Check sheet for the modelled part. Datum: model origin and axes. Units: mm. Face numbers are marked on the shaded views. Round coordinates to 2 decimals unless told otherwise and drop trailing zeros. Order: outer loops, then holes, each group sorted by start corner. A loop starts at its lowest first (then second) coordinate and runs counter-clockwise, first axis right, second up. Notation, with made-up numbers: (-39.5, -27.5) -> (15.5, -27.5) arc R16 ccw to (15.5, -2.5) -> close; hole circle Ø2 at (88.25, -34). An arc over 180 degrees is marked (long way). Use CSV: the item, a comma, the result in double quotes.
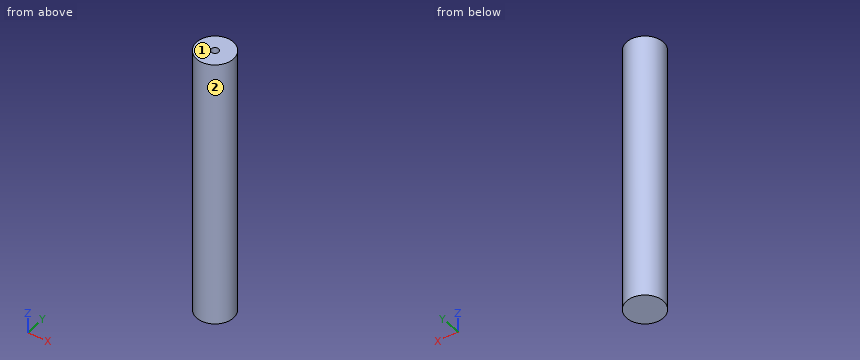
```python
from build123d import *

# Parameters (mm, degrees)
SKETCH009_R     = 5
PAD006_DEPTH    = 74
SKETCH010_R     = 1
POCKET002_DEPTH = 5
SKETCH011_R     = 1
POCKET003_DEPTH = 5


with BuildPart() as part:
    # Sketch009 → Pad006 (new body)
    with BuildSketch(Plane.XY):
        Circle(SKETCH009_R)
    extrude(amount=PAD006_DEPTH)

    # Sketch010 → Pocket002 (cut)
    with BuildSketch(Plane.XY):
        Circle(SKETCH010_R)
    extrude(amount=-POCKET002_DEPTH, mode=Mode.SUBTRACT)

    # Sketch011 (on Face4 of Pocket002) → Pocket003 (cut)
    with BuildSketch(Plane.XY.offset(74)):
        Circle(SKETCH011_R)
    extrude(amount=-POCKET003_DEPTH, mode=Mode.SUBTRACT)


solid = part.part
```
Q1. Sectioned sample at A-A, the plane y = -3. Enter the section's corners in (x, z), then the cut area to 3 significant figures.
Result sheet:
outline,"(-4, 0) -> (4, 0) -> (4, 74) -> (-4, 74) -> close"
area,"592 mm^2"
Q2. Sectioned sample at B-B, the plane x = 4.25. Enter the section's corners in (y, z).
Result sheet:
outline,"(-2.63, 0) -> (2.63, 0) -> (2.63, 74) -> (-2.63, 74) -> close"
Q3. Go/stop test with flat-tipped pins: pin 1 (5 mm diameter, centred on x = 2.5, z = 66, fed in from +Y); pin 2 (1 mm diameter, centred on y = 2.5, z = 45, fed in from -X); pin 3 (1.5 mm diameter, centred on x = 1, z = 46, fed in from -Y); pin 4 (1.8 mm diameter, centred on x = 0, y = 0, fed in from +Z). Record where each tip stops, or that it passes through.
Result sheet:
pin 1,"stops at y = 5"
pin 2,"stops at x = -4.58"
pin 3,"stops at y = -4.99"
pin 4,"stops at z = 69"
Q4. Mould release check, pull along X, two halves, no side actions. Record for the marked faces 1 and 2: pulls with the +X half, pulls with the -X half, needs draft (parallel to the pull), parting line crosses it, or undercut.
Result sheet:
face 1,"needs draft"
face 2,"parting line crosses it"
Q5. Sectioned sample at C-C, the plane z = 47.5. Enter the section's corners in (x, y), then the cut area to 3 significant figures.
Result sheet:
outline,"circle Ø10 at (0, 0)"
area,"78.5 mm^2"
Q6. Scan lines: L1, parallel to Y at x = 0, z = 71.45; L2, parallel to X at y = -0.25, z = 19; L3, parallel to X at y = -3.25, z = 34. Record each from-to range of solid material in increasing order.
Result sheet:
L1,"y = -5 to -1, 1 to 5"
L2,"x = -4.99 to 4.99"
L3,"x = -3.8 to 3.8"
